Build history of the part. All positions in model axes, mm. Round coordinates to 2 decimals unless told otherwise and drop trailing zeros. Write each loop counter-clockwise with the first axis right and the second up, starting at its lowest first coordinate (ties: lowest second). Pieces come first, ordered by that corner, then holes. Notation, with made-up numbers: (62.5, -39.75) -> (92.5, -39.75) arc R21 cw to (92.5, -7.75) -> close; hole circle Ø3 at (77, -17). An arc over 180 degrees is marked (long way). Answer in a Markdown table with one row per item. Add a question column.
from build123d import *

# Parameters (mm, degrees)
ESQUISSE1_W             = 32
ESQUISSE1_H             = 6
BOSS_EXTRU_1_DEPTH      = 3
ESQUISSE1_3_R           = 1.05
ENL_V_MAT_EXTRU_1_DEPTH = 19


with BuildPart() as part:
    # Esquisse1 → Boss.-Extru.1 (new body)
    with BuildSketch(Plane.XY):
        with Locations((-7.60481861, 2.703893443)):
            Rectangle(ESQUISSE1_W, ESQUISSE1_H)
    extrude(amount=BOSS_EXTRU_1_DEPTH)

    # Esquisse1_3 → Enl_v. mat.-Extru.1 (cut)
    with BuildSketch(Plane.XY):
        with BuildLine():
            ThreePointArc((2.39518139, 12.203893443), (-11.069395008, 21.584549624), (-15.204160687, 5.703893443))
            Line((-15.204160687, 5.703893443), (-0.005476534, 5.703893443))
            ThreePointArc((-0.005476534, 5.703893443), (1.77583757, 8.739317045), (2.39518139, 12.203893443))
        make_face()
        with BuildLine():
            Line((-0.005476534, 5.703893443), (-15.204160687, 5.703893443))
            ThreePointArc((-15.204160687, 5.703893443), (-7.60481861, 2.203893443), (-0.005476534, 5.703893443))
        make_face()
        with Locations((6.64518139, 2.703893443)):
            Circle(ESQUISSE1_3_R)
        with Locations(Location((-21.85481861, 2.703893443, 0), (0, 0, 180))):
            Circle(ESQUISSE1_3_R)
    extrude(amount=ENL_V_MAT_EXTRU_1_DEPTH, mode=Mode.SUBTRACT)


solid = part.part
(1) Saw through at A-A (z = 1.45). List the corners of the cut face in (x, y).
(2) Saw through at B-B (y = 5). List the corners of the cut face in (x, z).
(3) Drop a flat-ended pin along its axis: P1, Ø2.5, axis at x = 6.65, y = 2.7, coming from the -Z side. Give the stop position or say it passes through.
(4) Mould opens along X. For faces 1 (the face through (-7.726, 2.205, 1.479)), 2 (the face through (-8, -0.296, 1)), 3 (the face through (8.395, 3, 1)) say: pulls with the +X half, pulls with the -X half, needs draft (parallel to the pull), parting line crosses it, or undercut.
(5) Saw through at D-D (x = -11). List the corners of the cut face in (y, z).
(6) Saw through at C-C (x = -7). List the corners of the cut face in (y, z).
(7) Probe line 1 along X through (y, z) = (3.25, 0.4); line 2 along Y through (x, z) = (7.5, 0.5); line 3 along X through (y, z) = (2, 1.7). List the from-to ranges inside material, lowest first.
Answer sheet:
| question | item | result |
|---|---|---|
| 1 | outline | (-23.6, -0.3) -> (8.4, -0.3) -> (8.4, 5.7) -> (-0.01, 5.7) arc R10 cw to (-15.2, 5.7) -> (-23.6, 5.7) -> close; hole circle Ø2.1 at (-21.85, 2.7); hole circle Ø2.1 at (6.65, 2.7) |
| 2 | outline | (-23.6, 0) -> (-14.54, 0) -> (-14.54, 3) -> (-23.6, 3) -> close; (-0.67, 0) -> (8.4, 0) -> (8.4, 3) -> (-0.67, 3) -> close |
| 3 | P1 | stops at z = 0 |
| 4 | face 1 | undercut |
| 4 | face 2 | needs draft |
| 4 | face 3 | pulls with the +X half |
| 5 | outline | (-0.3, 0) -> (2.8, 0) -> (2.8, 3) -> (-0.3, 3) -> close |
| 6 | outline | (-0.3, 0) -> (2.22, 0) -> (2.22, 3) -> (-0.3, 3) -> close |
| 7 | line 1 | x = -23.6 to -22.75, -20.96 to -12.06, -3.15 to 5.75, 7.54 to 8.4 |
| 7 | line 2 | y = -0.3 to 2.09, 3.31 to 5.7 |
| 7 | line 3 | x = -23.6 to -22.63, -21.08 to 5.87, 7.42 to 8.4 |
